The drawing under review shows one solid part. Ordinate dimensions are in mm from its lowest x, y, z. A direction names the side the tool comes from. Coordinates: 2 decimals unless noted, no trailing zeros. Loops run counter-clockwise (first coordinate to the right, second up) from the corner with the lowest first, then second, coordinate; pieces in that order, holes last. Notation, with made-up numbers: (62.5, 29) -> (79.5, 29) arc R16 cw to (79.5, 40) -> close; hole circle Ø2 at (-5, -36). An arc over 180 degrees is marked (long way). Use a Markdown table: item, result.
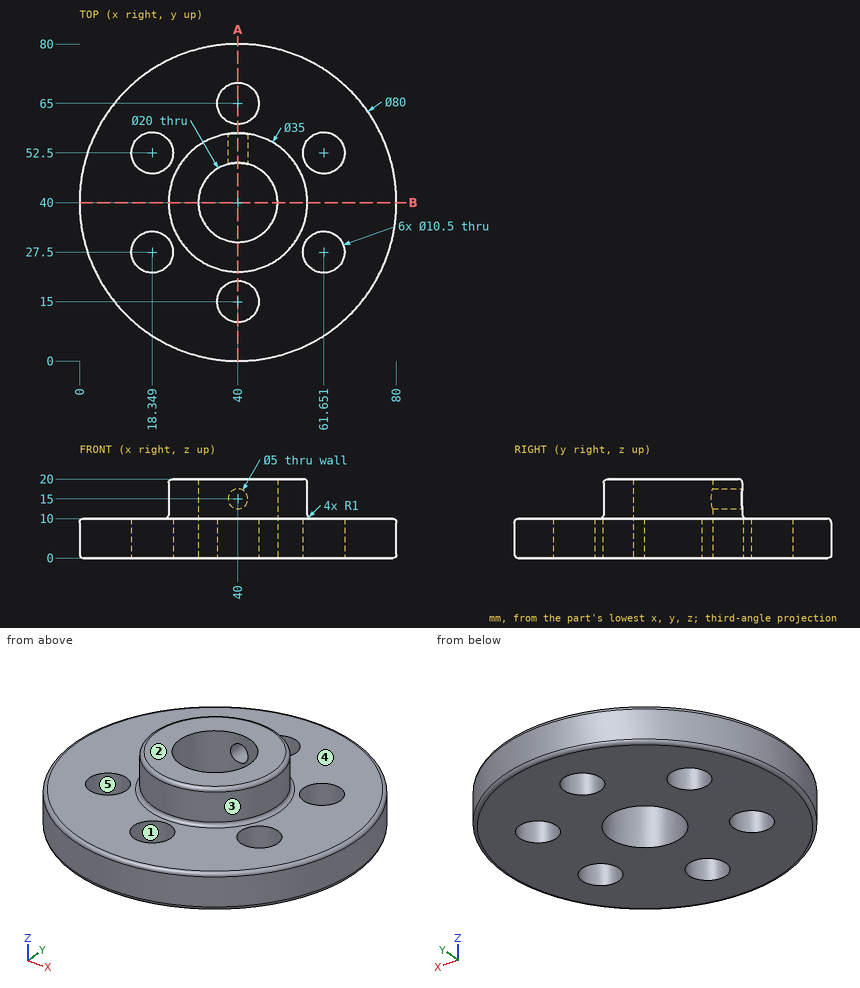
(1) Take a section at A-A on x = 40. State how many separate pieces and enclosed holes the cut face has.
Found:
| item | result |
|---|---|
| separate pieces | 5 |
| enclosed holes | 0 |
(2) Take a section at B-B on y = 40. Write out the cut boundary in (x, z), plus the area to 3 significant figures.
Found:
| item | result |
|---|---|
| outline | (0, 1) arc R1 ccw to (1, 0) -> (30, 0) -> (30, 20) -> (23.5, 20) arc R1 ccw to (22.5, 19) -> (22.5, 11) arc R1 cw to (21.5, 10) -> (1, 10) arc R1 ccw to (0, 9) -> close; (50, 0) -> (79, 0) arc R1 ccw to (80, 1) -> (80, 9) arc R1 ccw to (79, 10) -> (58.5, 10) arc R1 cw to (57.5, 11) -> (57.5, 19) arc R1 ccw to (56.5, 20) -> (50, 20) -> close |
| area | 749 mm^2 |
(3) Mouldability with a two-part tool opening along X and no side actions: class the marked faces 1, 2 and 3 as pulls with the +X half, pulls with the -X half, needs draft (parallel to the pull), parting line crosses it, or undercut.
Found:
| item | result |
|---|---|
| face 1 | undercut |
| face 2 | needs draft |
| face 3 | parting line crosses it |
(4) For line 1 along Z through (x, y) = (40, 52.25); line 2 along Y through (x, z) = (37.5, 9.5) (1 decimal); line 3 along Z through (x, y) = (66.5, 14), list the stretches that pass through material, from the lowest coordinate up.
Found:
| item | result |
|---|---|
| line 1 | z = 0 to 12.5, 17.5 to 20 |
| line 2 | y = 0.2 to 10.4, 19.6 to 30.3, 49.7 to 60.4, 69.6 to 79.8 |
| line 3 | z = 0 to 10 |
(5) For pin 1 Ø12 at (x, y) = (18.35, 52.5) entering from +Z; pin 2 Ø6.5 at (x, z) = (40, 15) entering from -Y; pin 3 Ø3 at (y, z) = (20.5, 13) entering from -X; pin 4 Ø12 at (x, z) = (24, 4.5) entering from +Y, all flat-tipped, find the tip position at first contact; note any pin that passes through.
Found:
| item | result |
|---|---|
| pin 1 | stops at z = 10 |
| pin 2 | stops at y = 22.5 |
| pin 3 | passes through |
| pin 4 | stops at y = 78.73 |
(6) For the marked faces 4 and 5, list the 3-axis set-ups (+Z, -Z, +X, -X, +Y, -Y) from which the entire face can be reached by the end or side of a thin tool; tool diameter is ignored.
Found:
| item | result |
|---|---|
| face 4 | +Z |
| face 5 | +Z, -Z |
